Here's how the part is built. I have some questions about the finished solid (model axes, mm). Face numbers are marked on the shaded views. Round coordinates to 2 decimals unless told otherwise and drop trailing zeros. Write each loop counter-clockwise with the first axis right and the second up, starting at its lowest first coordinate (ties: lowest second). Pieces come first, ordered by that corner, then holes. Notation, with made-up numbers: (-5, -32.75) - (35, -32.75) arc R16 cw to (35, -22.75) - close; hole circle Ø3 at (17, -33.75). An arc over 180 degrees is marked (long way). Use one line per item in the form item = value. Start each with the question number.
1. If I drill on line 1 along Y through (x, z) = (0, -5); line 2 along X through (y, z) = (9, -9); line 3 along Z through (x, y) = (33, -71.5), over which ranges is the centre line in solid material (lowest first)?
2. We'd pull the mould along X, two halves only. Please class the marked faces 1, 2 and 3: +X half, -X half, draft (parallel to the pull), parting line (faces both ways), or undercut.
3. I want a section at D-D, the plane z = 5.5. List the corners of the cut face in (x, y) for me.
4. I want a section at C-C, the plane z = -17.5. List the corners of the cut face in (x, y) for me, plus the area to 3 significant figures.
5. Will these pins go through, and if not, where does the flat tip stop? pin 1 (2 mm diameter, centred on x = 63.5, y = 87, fed in from -Z); pin 2 (1 mm diameter, centred on x = 39, y = -76, fed in from +Z); pin 3 (3 mm diameter, centred on x = -22.5, y = 100.5, fed in from -Z); pin 4 (5 mm diameter, centred on x = 78, z = 0, fed in from +Y).
6. I want a section at A-A, the plane x = 0. List the corners of the cut face in (y, z) for me, plus the area to 3 significant figures.
```python
from build123d import *


with BuildPart() as part:
    # Sketch1 → Revolve1 (revolve)
    with BuildSketch(Plane.YZ, mode=Mode.PRIVATE) as revolve1_sk:
        with BuildLine():
            ThreePointArc((-57.15, -39.5), (-43.428307314, -36.322800112), (-31.106422396, -29.5))
            Line((-31.106422396, -29.5), (-25.4, -29.5))
            Line((-25.4, -29.5), (-25.4, 2))
            Line((-25.4, 2), (-127, 10.888848214))
            Line((-127, 10.888848214), (-127, 8.881208539))
            Line((-127, 8.881208539), (-27.4, 0.167337652))
            Line((-27.4, 0.167337652), (-27.4, -23.683734158))
            ThreePointArc((-27.4, -23.683734158), (-41.079585236, -33.165904784), (-57.15, -37.5))
            Line((-57.15, -37.5), (-88.9, -37.5))
            Line((-88.9, -37.5), (-88.9, -39.5))
            Line((-88.9, -39.5), (-57.15, -39.5))
        make_face()
    revolve(revolve1_sk.sketch.rotate(Axis((0, 0, 14.051954895), (0, 0, -1)), 270), axis=Axis((0, 0, 14.051954895), (0, 0, -1)))


solid = part.part
```
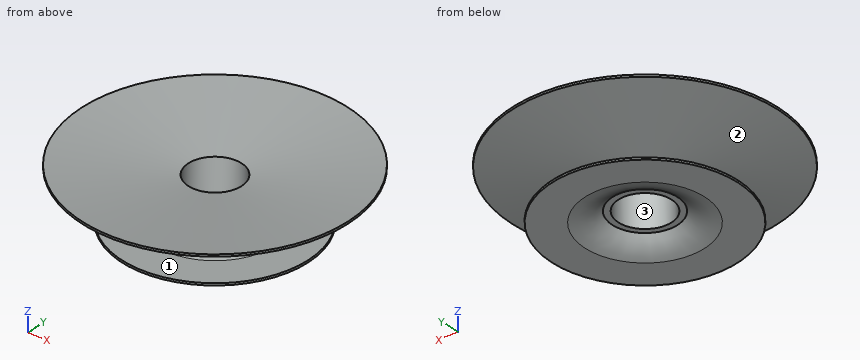
Model answer:
q1.line_1 = -27.4 to -25.4, 25.4 to 27.4
q1.line_2 = -25.88 to -23.75, 23.75 to 25.88
q1.line_3 = -39.5 to -37.5, 4.66 to 6.67
q2.face_1 = draft
q2.face_2 = parting line
q2.face_3 = undercut
q3.outline = circle Ø176.71 at (0, 0); hole circle Ø130.81 at (0, 0)
q4.outline = circle Ø54.8 at (0, 0); hole circle Ø50.8 at (0, 0)
q4.area = 332 mm2
q5.pin_1 = 7.11
q5.pin_2 = 7.3
q5.pin_3 = 6.65
q5.pin_4 = through
q6.outline = (-127, 8.88) - (-27.4, 0.17) - (-27.4, -23.68) arc R48.81 cw to (-57.15, -37.5) - (-88.9, -37.5) - (-88.9, -39.5) - (-57.15, -39.5) arc R50.8 ccw to (-31.11, -29.5) - (-25.4, -29.5) - (-25.4, 2) - (-127, 10.89) - close; (25.4, -29.5) - (31.11, -29.5) arc R50.8 ccw to (57.15, -39.5) - (88.9, -39.5) - (88.9, -37.5) - (57.15, -37.5) arc R48.81 cw to (27.4, -23.68) - (27.4, 0.17) - (127, 8.88) - (127, 10.89) - (25.4, 2) - close
q6.area = 797 mm2
